from build123d import *

# Parameters (mm, degrees)
F0_W         = 70
F0_H         = 80
F0_W_2       = 20.9936025798
F0_H_2       = 23.8757147082
F1_DEPTH     = 100
F2_W         = 41.873505339
F2_H         = 37.2992325574
F3_DEPTH     = 30
F4_R         = 6.4210037994
F5_DEPTH     = 50
F6_T1_DEPTH  = 85
F6_T3_DEPTH  = 95
F6_T5_DEPTH  = 115
F6_S9_W      = 10
F6_S9_H      = 10
F6_T10_DEPTH = 10


# Not quite as in the source:
# - a fillet or chamfer that OpenCascade refuses, or shapes differently, is made with other operations: its cross-section is extruded or revolved along the edge and cut away or added


with BuildPart() as f1:
    # F0 (on Top) → F1 (new body)
    with BuildSketch(Plane.XY):
        with Locations((-5.7970939631, 1.8514618278)):
            Rectangle(F0_W, F0_H)
        with Locations((9.6997073268, 13.7893191818)):
            Rectangle(F0_W_2, F0_H_2, mode=Mode.SUBTRACT)
    extrude(amount=F1_DEPTH)

    # F2 (on face) → F3 (join)
    with BuildSketch(Plane.XZ.offset(38.1485381722)):
        with Locations((-12.9710743204, 46.823351644)):
            Rectangle(F2_W, F2_H)
    extrude(amount=F3_DEPTH)

    # F4 (on face) → F5 (cut)
    with BuildSketch(Plane.XY.offset(65.4729679227)):
        with Locations((-24.8845424503, -53.2096363604)):
            Circle(F4_R)
    extrude(amount=-F5_DEPTH, mode=Mode.SUBTRACT)

    # F6: fillet of radius 10 on 3 edges, made by hand

    # F6_s2 → F6_t1 (cut)
    with BuildSketch(Plane.YZ.offset(-65.7970939631)):
        with BuildLine():
            ThreePointArc((-28.1485381722, 100), (-35.2196059841, 97.0710678119), (-38.1485381722, 90))
            Line((-38.1485381722, 90), (-38.1485381722, 100))
            Line((-38.1485381722, 100), (-28.1485381722, 100))
        make_face()
    extrude(amount=F6_T1_DEPTH, mode=Mode.SUBTRACT)

    # F6_s4 → F6_t3 (cut)
    with BuildSketch(Plane.XZ.offset(-66.8514618278)):
        with BuildLine():
            ThreePointArc((29.2029060369, 90), (26.2739738488, 97.0710678119), (19.2029060369, 100))
            Line((19.2029060369, 100), (29.2029060369, 100))
            Line((29.2029060369, 100), (29.2029060369, 90))
        make_face()
    extrude(amount=F6_T3_DEPTH, mode=Mode.SUBTRACT)

    # F6_s6 → F6_t5 (cut)
    with BuildSketch(Plane.XY.offset(-25)):
        with BuildLine():
            ThreePointArc((29.2029060369, -28.1485381722), (26.2739738488, -35.2196059841), (19.2029060369, -38.1485381722))
            Line((19.2029060369, -38.1485381722), (29.2029060369, -38.1485381722))
            Line((29.2029060369, -38.1485381722), (29.2029060369, -28.1485381722))
        make_face()
    extrude(amount=F6_T5_DEPTH, mode=Mode.SUBTRACT)


with BuildPart() as f6_tool8:
    # F6_s9 → F6_t10 (new body)
    with BuildSketch(Plane.YZ.offset(19.2029060369)):
        with Locations((-33.1485381722, 95)):
            Rectangle(F6_S9_W, F6_S9_H)
    extrude(amount=F6_T10_DEPTH)

    # F6_s11 → F6_t12 (revolve, cut)
    with BuildSketch(Plane(origin=(19.2029060369, -28.1485381722, 90), x_dir=(0, 0.7071067812, -0.7071067812), z_dir=(0, -0.7071067812, -0.7071067812))):
        with BuildLine():
            ThreePointArc((0, -10), (10, 0), (0, 10))
            Line((0, 10), (0, -10))
        make_face()
    revolve(axis=Axis((19.2029060369, -28.1485381722, 90), (1, 0, 0)), mode=Mode.SUBTRACT)


with BuildPart() as f1_1:
    add(f1.part)

    # F6_t7: cut F6_tool8
    add(f6_tool8.part, mode=Mode.SUBTRACT)


solid = f1_1.part
Could you check a few things on this model? Use its own coordinates, in mm. A direction names the side the tool comes from. Give positions to 0.01 mm unless a question says otherwise; leave off trailing zeros. Write each loop counter-clockwise with the first axis right and the second up, starting at its lowest first coordinate (ties: lowest second). Pieces come first, ordered by that corner, then holes. Notation, with made-up numbers: (-16.75, 71) - (-7.75, 71) arc R14 ccw to (-7.75, 75) - close; hole circle Ø6 at (66.25, -4). An arc over 180 degrees is marked (long way). Use CSV: the item, a comma, the result in double quotes. Start each with the question number.
Item 1: I'm going to push flat-ended pins straight in: pin 1 (24 mm diameter, centred on y = -55, z = 51.5, fed in from +X); pin 2 (8 mm diameter, centred on y = -53.5, z = 61.5, fed in from -X); pin 3 (15 mm diameter, centred on x = -24.88, y = -53.21, fed in from +Z); pin 4 (4 mm diameter, centred on x = -17, y = -3.5, fed in from -Z). Where does each tip first touch, or does it pass through?
Item 2: I want a section at D-D, the plane x = -12.5. Please give me the cut outline in (y, z), then the cut area to 3 significant figures.
Item 3: For faces 1 (the face through (-13, -53, 65.473)), 2 (the face through (-33.908, -53, 47)), 3 (the face through (20.197, 14, 49)), which set-ups out of +Z, -Z, +X, -X, +Y, -Y let a thin tool reach every point of the face, with its end or its side?
Item 4: I want a section at B-B, the plane z = 23.5. Please give me the cut outline in (x, y).
Item 5: I want a section at A-A, the plane x = 2.5. Please give me the cut outline in (y, z).
Item 6: If we mould it in two halves opening along Y, with no side actions, what happens to faces 4 (the face through (10, 1.851, 49)), 5 (the face through (-13, -68.149, 47)), 6 (the face through (-6, 41.851, 49)), 7 (the face through (-6, 2, 0))? For each: pulls with the +Y half, pulls with the -Y half, needs draft (parallel to the pull), parting line crosses it, or undercut.
Item 7: I want a section at C-C, the plane y = 5. Please give me the cut outline in (x, z).
Item 8: If I drill on line 1 along X through (y, z) = (11, 81); line 2 along Y through (x, z) = (16, 81); line 3 along Z through (x, y) = (-10, -52), over which ranges is the centre line in solid material (lowest first)?
Findings:
1,pin 1,"stops at x = 7.97"
1,pin 2,"stops at x = -33.91"
1,pin 3,"stops at z = 65.47"
1,pin 4,"stops at z = 0"
2,outline,"(-68.15, 28.17) - (-38.15, 28.17) - (-38.15, 0) - (41.85, 0) - (41.85, 100) - (-28.15, 100) arc R10 ccw to (-38.15, 90) - (-38.15, 65.47) - (-68.15, 65.47) - close"
2,area,"9,100 mm2"
3,face 1,"+Z, +X, -X, -Y"
3,face 2,"+Z, -Z, -X, -Y"
3,face 3,"+Z, -Z"
4,outline,"(-40.8, -38.15) - (19.2, -38.15) arc R10 ccw to (29.2, -28.15) - (29.2, 41.85) - (-40.8, 41.85) - close; hole (-0.8, 1.85) - (20.2, 1.85) - (20.2, 25.73) - (-0.8, 25.73) - close"
5,outline,"(-68.15, 28.17) - (-38.15, 28.17) - (-38.15, 0) - (1.85, 0) - (1.85, 100) - (-28.15, 100) arc R10 ccw to (-38.15, 90) - (-38.15, 65.47) - (-68.15, 65.47) - close; (25.73, 0) - (41.85, 0) - (41.85, 100) - (25.73, 100) - close"
6,face 4,"undercut"
6,face 5,"pulls with the -Y half"
6,face 6,"pulls with the +Y half"
6,face 7,"needs draft"
7,outline,"(-40.8, 0) - (-0.8, 0) - (-0.8, 100) - (-40.8, 100) - close; (20.2, 0) - (29.2, 0) - (29.2, 90) arc R10 ccw to (20.2, 99.95) - close"
8,line 1,"x = -40.8 to -0.8, 20.2 to 29.2"
8,line 2,"y = -38.15 to 1.85, 25.73 to 41.85"
8,line 3,"z = 28.17 to 65.47"
